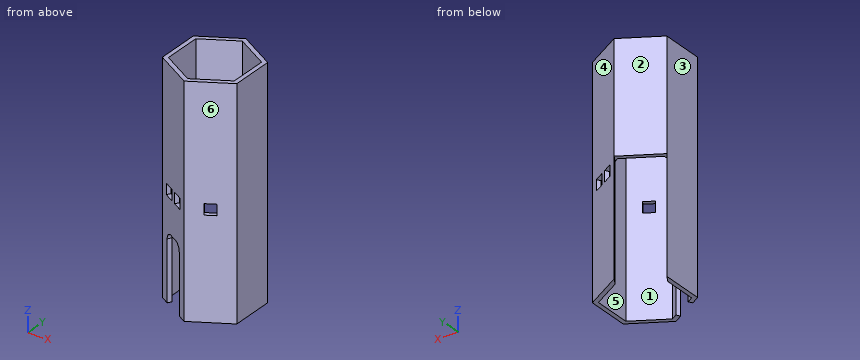
```python
from build123d import *

# Parameters (mm, degrees)
BOSS_EXTRUDE2_DEPTH = 940
CUT_EXTRUDE3_REACH  = 1020.577
SKETCH4_W           = 45
SKETCH4_H           = 45
CUT_EXTRUDE4_REACH  = 1020.577
SKETCH5_W           = 45
SKETCH5_H           = 45
CUT_EXTRUDE6_REACH  = 1020.577
SKETCH7_W           = 180
SKETCH7_H           = 480
SKETCH9_W           = 45
SKETCH9_H           = 45
CUT_EXTRUDE7_DEPTH  = 18


with BuildPart() as part:
    # Sketch1 → Boss-Extrude2 (new body)
    with BuildSketch(Plane.XY):
        Polygon((0, 180), (-155.884572681, 90), (-155.884572681, -90), (0, -180), (155.884572681, -90), (155.884572681, 90), align=None)
        Polygon((-137.884572681, 79.607695155), (-137.884572681, -79.607695155), (0, -159.215390309), (137.884572681, -79.607695155), (137.884572681, 79.607695155), (0, 159.215390309), align=None, mode=Mode.SUBTRACT)
    extrude(amount=BOSS_EXTRUDE2_DEPTH)

    # Sketch4 → Cut-Extrude3 (cut, up to next)
    with BuildSketch(Plane(origin=(77.942286341, -135, 0), x_dir=(0.8660254037844388, 0.4999999999999997, 0), z_dir=(0.4999999999999997, -0.8660254037844388, 0)), mode=Mode.PRIVATE) as cut_extrude3_sk1:
        with Locations((0, 442)):
            Rectangle(SKETCH4_W, SKETCH4_H)
    cut_extrude3_tool1 = extrude(cut_extrude3_sk1.sketch, amount=-CUT_EXTRUDE3_REACH, mode=Mode.PRIVATE) & part.part
    add(cut_extrude3_tool1.solids().sort_by_distance((77.942286, -135, 442))[0], mode=Mode.SUBTRACT)

    # Sketch5 → Cut-Extrude4 (cut, up to next)
    with BuildSketch(Plane(origin=(-77.942286341, -135, 0), x_dir=(0.8660254037844386, -0.5000000000000001, 0), z_dir=(-0.5000000000000001, -0.8660254037844386, 0)), mode=Mode.PRIVATE) as cut_extrude4_sk1:
        with Locations((34.5, 442)):
            Rectangle(SKETCH5_W, SKETCH5_H)
    cut_extrude4_tool1 = extrude(cut_extrude4_sk1.sketch, amount=-CUT_EXTRUDE4_REACH, mode=Mode.PRIVATE) & part.part
    # Sketch5 → Cut-Extrude4 (cut, up to next)
    with BuildSketch(Plane(origin=(-77.942286341, -135, 0), x_dir=(0.8660254037844386, -0.5000000000000001, 0), z_dir=(-0.5000000000000001, -0.8660254037844386, 0)), mode=Mode.PRIVATE) as cut_extrude4_sk2:
        with Locations((-34.5, 442)):
            Rectangle(SKETCH5_W, SKETCH5_H)
    cut_extrude4_tool2 = extrude(cut_extrude4_sk2.sketch, amount=-CUT_EXTRUDE4_REACH, mode=Mode.PRIVATE) & part.part
    # Sketch5 → Cut-Extrude4 (cut, up to next)
    with BuildSketch(Plane(origin=(-77.942286341, -135, 0), x_dir=(0.8660254037844386, -0.5000000000000001, 0), z_dir=(-0.5000000000000001, -0.8660254037844386, 0)), mode=Mode.PRIVATE) as cut_extrude4_sk3:
        with BuildLine():
            Line((-20, 280), (20, 280))
            ThreePointArc((20, 280), (41.213203436, 271.213203436), (50, 250))
            Line((50, 250), (50, 0))
            Line((50, 0), (-50, 0))
            Line((-50, 0), (-50, 250))
            ThreePointArc((-50, 250), (-41.213203436, 271.213203436), (-20, 280))
        make_face()
    cut_extrude4_tool3 = extrude(cut_extrude4_sk3.sketch, amount=-CUT_EXTRUDE4_REACH, mode=Mode.PRIVATE) & part.part
    add(cut_extrude4_tool1.solids().sort_by_distance((-48.06441, -152.25, 442))[0], mode=Mode.SUBTRACT)
    add(cut_extrude4_tool2.solids().sort_by_distance((-107.820163, -117.75, 442))[0], mode=Mode.SUBTRACT)
    add(cut_extrude4_tool3.solids().sort_by_distance((-77.942286, -135, 138.135305))[0], mode=Mode.SUBTRACT)

    # Sketch7 → Cut-Extrude6 (cut, up to next)
    with BuildSketch(Plane(origin=(-77.942286341, 135, 0), x_dir=(0.8660254037844388, 0.49999999999999983, 0), z_dir=(-0.4999999999999998, 0.8660254037844387, 0)), mode=Mode.PRIVATE) as cut_extrude6_sk1:
        with Locations((0, -240)):
            Rectangle(SKETCH7_W, SKETCH7_H)
    cut_extrude6_tool1 = extrude(cut_extrude6_sk1.sketch, amount=-CUT_EXTRUDE6_REACH, mode=Mode.PRIVATE) & part.part
    add(cut_extrude6_tool1.solids().sort_by_distance((-77.942286, 135, 240))[0], mode=Mode.SUBTRACT)

    # Sketch9 → Cut-Extrude7 (cut)
    with BuildSketch(Plane(origin=(77.942286341, 135, 0), x_dir=(0.8660254037844386, -0.4999999999999999, 0), z_dir=(0.49999999999999994, 0.8660254037844387, 0))):
        with Locations((-34.5, -442)):
            Rectangle(SKETCH9_W, SKETCH9_H)
        with Locations((34.5, -442)):
            Rectangle(SKETCH9_W, SKETCH9_H)
    extrude(amount=-CUT_EXTRUDE7_DEPTH, mode=Mode.SUBTRACT)


solid = part.part
```
Read the model definition and answer for the solid it produces. Units are mm, in the model's axes. Face numbers are marked on the shaded views. A direction names the side the tool comes from. Coordinates: 2 decimals unless noted, no trailing zeros. Loops run counter-clockwise (first coordinate to the right, second up) from the corner with the lowest first, then second, coordinate; pieces in that order, holes last.
(1) The part is cut by section D-D (z = 335.5). Determine the outline of the cut face in (x, y), and give its area (3 significant figures).
Solution:
outline: (-155.88, -90) - (0, -180) - (155.88, -90) - (155.88, 90) - (0, 180) - (18, 148.82) - (137.88, 79.61) - (137.88, -79.61) - (0, -159.22) - (-137.88, -79.61) - (-137.88, 58.82) - (-155.88, 90) - close
area: 14,900 mm2
(2) The part is cut by section B-B (y = 22). Determine the outline of the cut face in (x, z), and give its area (3 significant figures).
Solution:
outline: (-155.88, 0) - (-137.88, 0) - (-137.88, 940) - (-155.88, 940) - close; (137.88, 0) - (155.88, 0) - (155.88, 940) - (137.88, 940) - close
area: 33,800 mm2
(3) A tool of negligible diameter and unlimited length cuts with its end or side. For the marked faces 1 and 2, from which of +Z, -Z, +X, -X, +Y, -Y can it reach the whole face along a straight path? Write none if from no direction.
Solution:
face 1: +Z, -Z
face 2: +Z, -Z, -X, +Y
(4) Flat-ended cylindrical pins translate along their axes: pin 1 Ø2 at (y, z) = (126.5, 719.5) entering from +X; pin 2 Ø18 at (x, y) = (-75, -133.5) entering from -Z; pin 3 Ø19 at (x, y) = (46, 148.5) entering from -Z; pin 4 Ø11.5 at (x, y) = (-55, -148.5) entering from -Z. Find the tip coordinate at first contact, or state that the pin passes through.
Solution:
pin 1: stops at x = 94.4
pin 2: stops at z = 280
pin 3: stops at z = 0
pin 4: stops at z = 277.33
(5) Consider line 1 along X through (y, z) = (-42.5, 616); line 2 along X through (y, z) = (75, 78); line 3 along Y through (x, z) = (-128.5, 642.5). Determine where each line is inside the solid, lowest interval first.
Solution:
line 1: x = -155.88 to -137.88, 137.88 to 155.88
line 2: x = -155.88 to -147.22, 137.88 to 155.88
line 3: y = -105.81 to -85.03, 85.03 to 105.81
(6) The part is cut by section A-A (z = 748.5). Determine the outline of the cut face in (x, y), and give its area (3 significant figures).
Solution:
outline: (-155.88, -90) - (0, -180) - (155.88, -90) - (155.88, 90) - (0, 180) - (-155.88, 90) - close; hole (-137.88, -79.61) - (0, -159.22) - (137.88, -79.61) - (137.88, 79.61) - (0, 159.22) - (-137.88, 79.61) - close
area: 18,300 mm2
(7) The part is cut by section C-C (z = 129). Determine the outline of the cut face in (x, y), and give its area (3 significant figures).
Solution:
outline: (-155.88, -90) - (-121.24, -110) - (-112.24, -94.41) - (-137.88, -79.61) - (-137.88, 58.82) - (-155.88, 90) - close; (-34.64, -160) - (0, -180) - (155.88, -90) - (155.88, 90) - (0, 180) - (18, 148.82) - (137.88, 79.61) - (137.88, -79.61) - (0, -159.22) - (-25.64, -144.41) - close
area: 13,100 mm2
(8) The mould has two halves that part along Y. Classify the marked faces 3, 4, 5 and 6: released by +Y, released by -Y, zero draft, split by the parting line, or undercut.
Solution:
face 3: zero draft
face 4: released by +Y
face 5: undercut
face 6: released by -Y
